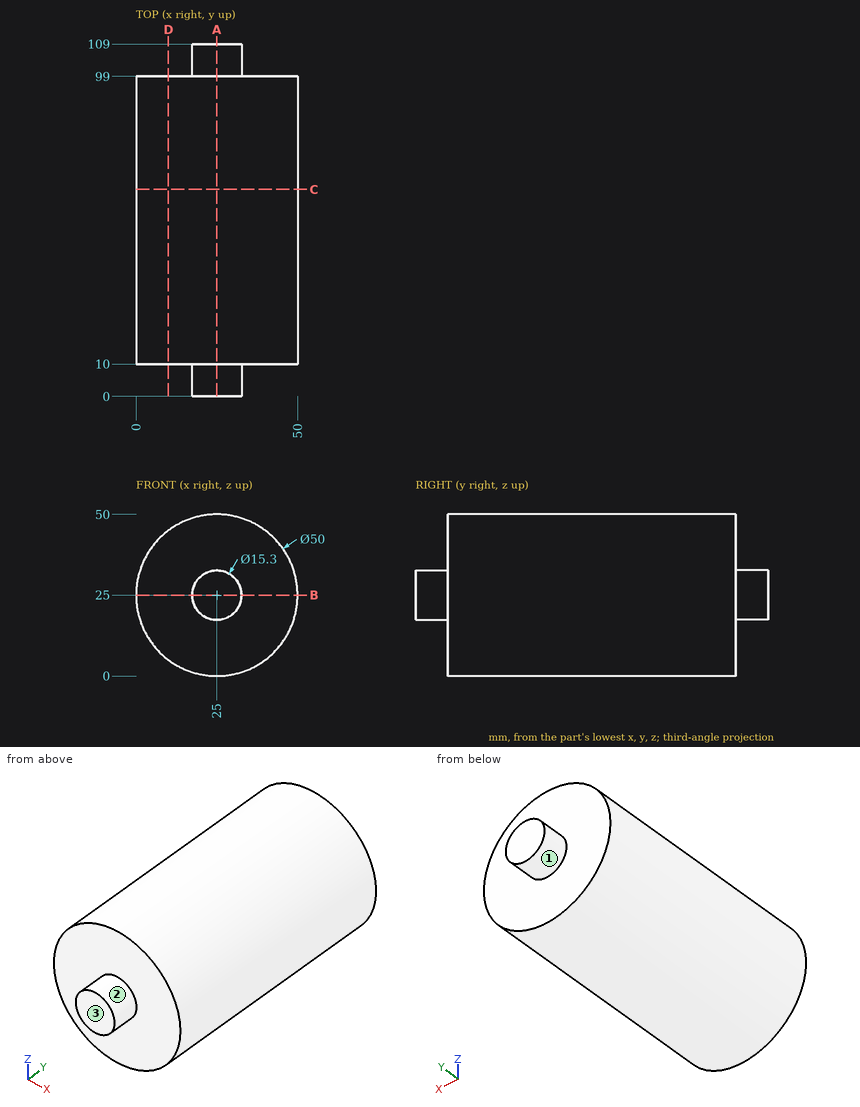
Input: dimensioned drawing with shaded views. Units: mm. Origin: part minimum x, y, z. A direction names the side the tool comes from. Give positions to 0.01 mm unless a question says otherwise; leave off trailing zeros. Loops run counter-clockwise (first coordinate to the right, second up) from the corner with the lowest first, then second, coordinate; pieces in that order, holes last. Notation, with made-up numbers: (22.25, 80.5) -> (69.25, 80.5) arc R16 ccw to (69.25, 96.5) -> close; hole circle Ø1 at (54.5, 10). An arc over 180 degrees is marked (long way). Use a Markdown table: item, result.
Q1. First-contact query: P1, Ø10, axis at x = 20, y = 77.5, coming from the +Z side; P2, Ø2, axis at x = 35, y = 83, coming from the -Z side; P3, Ø10, axis at x = 11.5, z = 16, coming from the -Y side. Flat tips, straight axial feed; report the tip coordinate or a pass-through.
Entries:
| item | result |
|---|---|
| P1 | stops at z = 50 |
| P2 | stops at z = 1.68 |
| P3 | stops at y = 10 |
Q2. Section query B-B, the plane z = 25. Return the cut outline in (x, y).
Entries:
| item | result |
|---|---|
| outline | (0, 10) -> (17.35, 10) -> (17.35, 0) -> (32.65, 0) -> (32.65, 10) -> (50, 10) -> (50, 99) -> (32.65, 99) -> (32.65, 109) -> (17.35, 109) -> (17.35, 99) -> (0, 99) -> close |
Q3. Ray query, probe 1 along Y at (x, z) = (45, 22); probe 2 along Z at (x, y) = (47, 42.5); probe 3 along Z at (x, y) = (18.5, 99.5). Return the intervals inside material, ascending. Write a range as from..to.
Entries:
| item | result |
|---|---|
| probe 1 | y = 10..99 |
| probe 2 | z = 13.13..36.87 |
| probe 3 | z = 20.97..29.03 |
Q4. Section query A-A, the plane x = 25. Return the cut outline in (y, z).
Entries:
| item | result |
|---|---|
| outline | (0, 17.35) -> (10, 17.35) -> (10, 0) -> (99, 0) -> (99, 17.35) -> (109, 17.35) -> (109, 32.65) -> (99, 32.65) -> (99, 50) -> (10, 50) -> (10, 32.65) -> (0, 32.65) -> close |
Q5. Section query D-D, the plane x = 10. Return the cut outline in (y, z).
Entries:
| item | result |
|---|---|
| outline | (10, 5) -> (99, 5) -> (99, 45) -> (10, 45) -> close |
Q6. Section query C-C, the plane y = 64. Return the cut outline in (x, z), plus the area to 3 significant figures.
Entries:
| item | result |
|---|---|
| outline | circle Ø50 at (25, 25) |
| area | 1,960 mm² |
Q7. Access query for the marked faces 1, 2 and 3. Directions: +Z, -Z, +X, -X, +Y, -Y. A direction counts if a zero-diameter tool reaches every point of the face in a straight line with its end or side. Return the directions, or none.
Entries:
| item | result |
|---|---|
| face 1 | +Y |
| face 2 | -Y |
| face 3 | +Z, -Z, +X, -X, -Y |
